The model under review builds one solid part; all positions refer to its coordinate system, in mm. A direction names the side the tool comes from. Give positions to 0.01 mm unless a question says otherwise; leave off trailing zeros. Order: outer loops, then holes, each group sorted by start corner. A loop starts at its lowest first (then second) coordinate and runs counter-clockwise, first axis right, second up. Notation, with made-up numbers: (79.5, -5) - (95.5, -5) arc R25 ccw to (95.5, 10) - close; hole circle Ø9 at (48, 51.5). An arc over 180 degrees is marked (long way). Use CSV: the item, a comma, the result in double quotes.
```python
from build123d import *

# Parameters (mm, degrees)
BOSS_EXTRUDE1_DEPTH  = 5.334
FUSELAGE_SLOTS_REACH = 7.334
RUDDER_SLOT_REACH    = 7.334
SKETCH4_W            = 25.4
SKETCH4_H            = 5.334


with BuildPart() as part:
    # Sketch1 → Boss-Extrude1 (new body)
    with BuildSketch(Plane(origin=(0, 0, 0), x_dir=(1, 0, 0), z_dir=(0, 1, 0))):
        with BuildLine():
            Line((15.970216498, 123.888067637), (0, 0))
            Line((0, 0), (15.970216498, -123.888067637))
            add(Edge.make_bspline(
                [(15.970216498, -123.888067637), (16.496348793, -127.969509697), (20.974883006, -132.098944904), (26.457102776, -133.85926391), (28.727885995, -134.31821318)],
                knots=[0, 0, 0, 0, 0.137873605, 0.230135461, 0.230135461, 0.230135461, 0.230135461], degree=3))
            Line((28.727885995, -134.31821318), (58.856137193, -114.786657988))
            Line((58.856137193, -114.786657988), (58.856137193, 114.786657988))
            Line((58.856137193, 114.786657988), (28.727885995, 134.31821318))
            add(Edge.make_bspline(
                [(15.970216498, 123.888067637), (16.496348793, 127.969509697), (20.974883006, 132.098944904), (26.457102776, 133.85926391), (28.727885995, 134.31821318)],
                knots=[0, 0, 0, 0, 0.137873605, 0.230135461, 0.230135461, 0.230135461, 0.230135461], degree=3))
        make_face()
        with BuildLine():
            add(Edge.make_bspline(
                [(28.727885995, 134.31821318), (31.449320367, 134.868243807), (36.288781724, 135.203179668), (46.054708275, 135.145094132), (57.878857589, 134.457454778), (71.986589127, 133.257487146), (78.619292876, 126.55856753), (81.681846945, 123.009151118), (81.805097467, 121.83833135)],
                knots=[0.230135461, 0.230135461, 0.230135461, 0.230135461, 0.340707261, 0.419473129, 0.623495844, 0.825009795, 0.952423895, 1, 1, 1, 1], degree=3))
            Line((28.727885995, 134.31821318), (58.856137193, 114.786657988))
            Line((58.856137193, 114.786657988), (58.856137193, -114.786657988))
            Line((58.856137193, -114.786657988), (28.727885995, -134.31821318))
            add(Edge.make_bspline(
                [(28.727885995, -134.31821318), (31.449320367, -134.868243807), (36.288781724, -135.203179668), (46.054708275, -135.145094132), (57.878857589, -134.457454778), (71.986589127, -133.257487146), (78.619292876, -126.55856753), (81.681846945, -123.009151118), (81.805097467, -121.83833135)],
                knots=[0.230135461, 0.230135461, 0.230135461, 0.230135461, 0.340707261, 0.419473129, 0.623495844, 0.825009795, 0.952423895, 1, 1, 1, 1], degree=3))
            Line((81.805097467, -121.83833135), (91.952571506, -25.442283053))
            Line((91.952571506, -25.442283053), (69.447862014, -4.983456242))
            Line((69.447862014, -4.983456242), (69.447862014, 4.983456242))
            Line((69.447862014, 4.983456242), (91.952571506, 25.442283053))
            Line((91.952571506, 25.442283053), (81.805097467, 121.83833135))
        make_face()
    extrude(amount=BOSS_EXTRUDE1_DEPTH)

    # Sketch3 → Fuselage Slots (cut, up to next)
    with BuildSketch(Plane(origin=(0, 5.334, 0), x_dir=(1, 0, 0), z_dir=(0, 1, 0)), mode=Mode.PRIVATE) as fuselage_slots_sk1:
        Polygon((50.911526431, 9.044666188), (25.571689625, 10.791855537), (25.204779861, 5.470489808), (50.544616668, 3.723300459), align=None)
    fuselage_slots_tool1 = extrude(fuselage_slots_sk1.sketch, amount=-FUSELAGE_SLOTS_REACH, mode=Mode.PRIVATE) & part.part
    add(fuselage_slots_tool1.solids().sort_by_distance((38.058153, 5.334, -7.257578))[0], mode=Mode.SUBTRACT)
    # Sketch3 → Fuselage Slots (cut, up to next)
    with BuildSketch(Plane(origin=(0, 5.334, 0), x_dir=(1, 0, 0), z_dir=(0, 1, 0)), mode=Mode.PRIVATE) as fuselage_slots_sk2:
        Polygon((25.571689625, -10.791855537), (50.911526431, -9.044666188), (50.544616668, -3.723300459), (25.204779861, -5.470489808), align=None)
    fuselage_slots_tool2 = extrude(fuselage_slots_sk2.sketch, amount=-FUSELAGE_SLOTS_REACH, mode=Mode.PRIVATE) & part.part
    add(fuselage_slots_tool2.solids().sort_by_distance((38.058153, 5.334, 7.257578))[0], mode=Mode.SUBTRACT)

    # Sketch4 → Rudder Slot (cut, up to next)
    with BuildSketch(Plane(origin=(0, 5.334, 0), x_dir=(1, 0, 0), z_dir=(0, 1, 0)), mode=Mode.PRIVATE) as rudder_slot_sk1:
        with Locations((17.78, 0)):
            Rectangle(SKETCH4_W, SKETCH4_H)
    rudder_slot_tool1 = extrude(rudder_slot_sk1.sketch, amount=-RUDDER_SLOT_REACH, mode=Mode.PRIVATE) & part.part
    add(rudder_slot_tool1.solids().sort_by_distance((17.78, 5.334, 0))[0], mode=Mode.SUBTRACT)


solid = part.part
```
Item 1: Clearance check with flat-ended pins moving along their axes: pin 1 (1.6 mm diameter, centred on y = 2, z = 1, fed in from +X); pin 2 (3 mm diameter, centred on x = 56.5, y = 3, fed in from -Z); pin 3 (2 mm diameter, centred on y = 3, z = 34.5, fed in from -X). State where each tip first meets the part, or that it passes through.
Results list:
pin 1,"stops at x = 69.45"
pin 2,"stops at z = -134.59"
pin 3,"stops at x = 4.32"
Item 2: Mouldability with a two-part tool opening along X and no side actions: class faces 4 (the face through (37.7, 2.7, -4.61)), 5 (the face through (86.95, 2.63, -72.97)), 6 (the face through (7.873, 2.63, 61.077)), 7 (the face through (45, 0, -2)) as pulls with the +X half, pulls with the -X half, needs draft (parallel to the pull), parting line crosses it, or undercut.
Results list:
face 4,"undercut"
face 5,"pulls with the +X half"
face 6,"pulls with the -X half"
face 7,"needs draft"
Item 3: Take a section at C-C, the plane z = -85.5. Give the boundary of the cut face in (x, y), and give its area (3 significant figures).
Results list:
outline,"(11.02, 0) - (85.63, 0) - (85.63, 5.33) - (11.02, 5.33) - close"
area,"398 mm2"
Item 4: Take a section at D-D, the plane z = -28. Give the boundary of the cut face in (x, y).
Results list:
outline,"(3.61, 0) - (91.68, 0) - (91.68, 5.33) - (3.61, 5.33) - close"
Item 5: Take a section at A-A, the plane y = 1.8. State how many separate pieces and enclosed holes the cut face has, and give its area (3 significant figures).
Results list:
separate pieces,"1"
enclosed holes,"3"
area,"19,900 mm2"
Item 6: Wall thickness on L1, parallel to Z at x = 40, y = 2.45; L2, parallel to Z at x = 41, y = 3.8; L3, parallel to Z at x = 26.5, y = 0.45: over which ranges is each line inside the solid? List them lowest first.
Results list:
L1,"z = -135.17 to -9.8, -4.45 to 4.45, 9.8 to 135.17"
L2,"z = -135.16 to -9.73, -4.38 to 4.38, 9.73 to 135.16"
L3,"z = -133.78 to -10.73, -5.38 to -2.67, 2.67 to 5.38, 10.73 to 133.78"
Item 7: Tool access review of faces 1 (the face through (30.48, 3, 0)), 2 (the face through (86.808, 2.63, 74.315)), 3 (the face through (69.448, 3, 0)): name each direction out of +Z, -Z, +X, -X, +Y, -Y from which nothing blocks a thin tool from reaching the whole face with its end or side.
Results list:
face 1,"+Y, -Y"
face 2,"+Z, +X, +Y, -Y"
face 3,"+X, +Y, -Y"
